Source: CAD feature listing. Evaluate the final solid. Frame: model axes, mm. Face numbers are marked on the shaded views. A direction names the side the tool comes from. Round coordinates to 2 decimals unless told otherwise and drop trailing zeros. Loops run counter-clockwise (first coordinate to the right, second up) from the corner with the lowest first, then second, coordinate; pieces in that order, holes last. Notation, with made-up numbers: (41, 89) -> (71, 89) arc R27 cw to (71, 125) -> close; hole circle Ø5 at (79, 42). An arc over 180 degrees is marked (long way). Write item = value, one per line.
from build123d import *

# Parameters (mm, degrees)
SKETCH_R     = 15
PAD_DEPTH    = 35.98
SKETCH001_R  = 15
PAD001_DEPTH = 40
POCKET_DEPTH = 45
FILLET_R     = 4


with BuildPart() as part:
    # Sketch → Pad (new body)
    with BuildSketch(Plane.XY):
        with BuildLine():
            ThreePointArc((-16.5, 25.05494), (0, -30), (16.5, 25.05494))
            Line((16.5, 25.05494), (16.5, 120))
            Line((16.5, 120), (-16.5, 120))
            Line((-16.5, 120), (-16.5, 25.05494))
        make_face()
        Circle(SKETCH_R, mode=Mode.SUBTRACT)
    extrude(amount=PAD_DEPTH)

    # Sketch001 (on Face3 of Pad) → Pad001 (join)
    with BuildSketch(Plane(origin=(0, 120, 0), x_dir=(-1, 0, 0), z_dir=(0, 1, 0))):
        with Locations((0, 17.99)):
            Circle(SKETCH001_R)
    extrude(amount=PAD001_DEPTH)

    # Sketch002 (on Face6 of Pad001) → Pocket (cut)
    with BuildSketch(Plane(origin=(0, 120, 0), x_dir=(-1, 0, 0), z_dir=(0, 1, 0))):
        Polygon((-16.5, 35.98), (-16.5, 28.908932), (-9.428932, 35.98), align=None)
        Polygon((16.5, 35.98), (16.5, 28.908932), (9.428932, 35.98), align=None)
        Polygon((16.5, 0), (9.428932, 0), (16.5, 7.071068), align=None)
        Polygon((-16.5, 0), (-9.428932, 0), (-16.5, 7.071068), align=None)
    extrude(amount=-POCKET_DEPTH, mode=Mode.SUBTRACT)

    # Fillet
    fillet_edges = [part.edges().sort_by_distance(p)[0] for p in [
        (-12.964466, 75, 3.535534),
        (-12.964466, 75, 32.444466),
        (12.964466, 75, 32.444466),
        (12.964466, 75, 3.535534),
    ]]
    fillet(fillet_edges, radius=FILLET_R)


solid = part.part
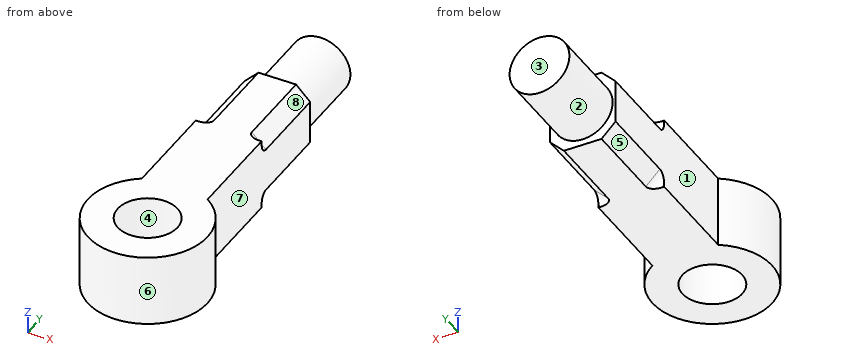
1. Set-up query: the marked faces 5, 6, 7 and 8. Return all of +Z, -Z, +X, -X, +Y, -Y with unobstructed straight access to the full face (end or side cutting, diameter ignored); none if empty.
Evaluation:
face_5 = -Z, -X, +Y
face_6 = +Z, -Z
face_7 = +Z, -Z, +X, +Y
face_8 = +Z, +X, +Y
2. Section query D-D (y = 108). Return the cut outline in (x, z), then the cut area to 3 significant figures.
Evaluation:
outline = (-16.5, 7.07) -> (-9.43, 0) -> (9.43, 0) -> (16.5, 7.07) -> (16.5, 28.91) -> (9.43, 35.98) -> (-9.43, 35.98) -> (-16.5, 28.91) -> close
area = 1,090 mm²
3. Section query A-A (y = 0). Return the cut outline in (x, z), then the cut area to 3 significant figures.
Evaluation:
outline = (-30, 0) -> (-15, 0) -> (-15, 35.98) -> (-30, 35.98) -> close; (15, 0) -> (30, 0) -> (30, 35.98) -> (15, 35.98) -> close
area = 1,080 mm²
4. Contact query for flat-ended pins moving along their axis: pin 1 Ø1.6 at (x, z) = (-15.5, 0.5) entering from +Y; pin 2 Ø8 at (x, y) = (1.5, 52) entering from -Z; pin 3 Ø1 at (y, z) = (120, 11) entering from +X; pin 4 Ø4 at (x, z) = (23.5, 24) entering from -Y. Output: stop coordinate, or through.
Evaluation:
pin_1 = 75.09
pin_2 = 0
pin_3 = 16.5
pin_4 = -20.92
5. Section query C-C (z = 17.99). Return the cut outline in (x, y), then the cut area to 3 significant figures.
Evaluation:
outline = (-16.5, 25.05) arc R30 ccw (long way) to (16.5, 25.05) -> (16.5, 120) -> (15, 120) -> (15, 160) -> (-15, 160) -> (-15, 120) -> (-16.5, 120) -> close; hole circle Ø30 at (0, 0)
area = 6,340 mm²
6. Line query: probe 1 along Y at (x, z) = (0, 10); probe 2 along Y at (x, z) = (-10, 16); probe 3 along X at (y, z) = (54, 13). Output: solid intervals per line, ascending. Write a range as from..to.
Evaluation:
probe_1 = -30..-15, 15..160
probe_2 = -28.28..-11.18, 11.18..160
probe_3 = -16.5..16.5
7. Section query B-B (x = 0). Return the cut outline in (y, z), then the cut area to 3 significant figures.
Evaluation:
outline = (-30, 0) -> (-15, 0) -> (-15, 35.98) -> (-30, 35.98) -> close; (15, 0) -> (120, 0) -> (120, 2.99) -> (160, 2.99) -> (160, 32.99) -> (120, 32.99) -> (120, 35.98) -> (15, 35.98) -> close
area = 5,520 mm²
8. Mould query, pull axis X, two halves, no side actions, for the marked faces 1, 2, 3 and 4. Classes: released by +X, released by -X, zero draft, split by the parting line, or undercut.
Evaluation:
face_1 = released by -X
face_2 = split by the parting line
face_3 = zero draft
face_4 = undercut
